Source: CAD feature listing. Evaluate the final solid. Frame: model axes, mm. A direction names the side the tool comes from. Coordinates: 2 decimals unless noted, no trailing zeros. Write each loop counter-clockwise with the first axis right and the second up, starting at its lowest first coordinate (ties: lowest second). Pieces come first, ordered by that corner, then holes. Notation, with made-up numbers: (-13.5, 45) -> (23.5, 45) arc R26 ccw to (23.5, 60) -> close; hole circle Ø2 at (17.5, 11.25). An arc over 180 degrees is marked (long way). One line per item, written item: value. Start each with the question number.
1. First-contact query: P1, Ø3, axis at x = -13, y = -54.5, coming from the -Z side; P2, Ø8.5, axis at y = -38, z = -12.5, coming from the +X side; P3, Ø6, axis at y = -34.5, z = -4, coming from the +X side. Flat tips, straight axial feed; report the tip coordinate or a pass-through.
2. Access query for faces 3 (the cylindrical face through (-32.22, -31.29, 0.51)), 4 (the flat face through (-29, -56.5, -8)). Directions: +Z, -Z, +X, -X, +Y, -Y. A direction counts if a zero-diameter tool reaches every point of the face in a straight line with its end or side. Return the directions, or none.
3. Mould query, pull axis X, two halves, no side actions, for faces 1 (the flat face through (-29, 1, -17)), 2 (the cylindrical face through (-0.86, -55.6, -8.62)). Classes: released by +X, released by -X, zero draft, split by the parting line, or undercut.
4. Line query: line 1 (Y direction, x = -28.25, z = 0.55); line 2 (Z direction, x = -35, y = -31); line 3 (X direction, y = -18, z = -9.25). Output: solid intervals per line, ascending.
5. Section query D-D, the plane x = -51.5. Output: boundary loops of the cut face in (y, z), and give its area (3 significant figures).
6. Section query C-C, the plane y = -55.5. Output: boundary loops of the cut face in (x, z), and give its area (3 significant figures).
7. Section query B-B, the plane z = -1. Output: boundary loops of the cut face in (x, y).
8. Section query A-A, the plane x = -28.25. Output: boundary loops of the cut face in (y, z).
from build123d import *

# Parameters (mm, degrees)
F0_W     = 60
F0_H     = 60
F0_W_2   = 56.5
F0_H_2   = 56.5
F1_DEPTH = 17
F2_DEPTH = 1
F3_DEPTH = 17
F4_R     = 5
F5_DEPTH = 25
F6_R     = 3


with BuildPart() as f1:
    # F0 (on Top) → F1 (new body)
    with BuildSketch(Plane.XY):
        with Locations((-28.25, -28.25)):
            Rectangle(F0_W, F0_H)
        with Locations((-28.25, -28.25)):
            Rectangle(F0_W_2, F0_H_2, mode=Mode.SUBTRACT)
    extrude(amount=-F1_DEPTH)

    # F0 (on Top) → F2 (join)
    with BuildSketch(Plane.XY):
        with Locations((-28.25, -28.25)):
            Rectangle(F0_W, F0_H)
        with Locations((-28.25, -28.25)):
            Rectangle(F0_W_2, F0_H_2, mode=Mode.SUBTRACT)
        with BuildLine():
            ThreePointArc((1.75, 1.75), (-28.25, 14.176407), (-58.25, 1.75))
            Line((-58.25, 1.75), (1.75, 1.75))
        make_face()
        with BuildLine():
            Line((1.75, 1.75), (1.75, -58.25))
            ThreePointArc((1.75, -58.25), (10.946889, -44.485883), (14.176407, -28.25))
            ThreePointArc((14.176407, -28.25), (10.946889, -12.014117), (1.75, 1.75))
        make_face()
        with BuildLine():
            Line((1.75, -58.25), (-58.25, -58.25))
            ThreePointArc((-58.25, -58.25), (-28.25, -70.676407), (1.75, -58.25))
        make_face()
        with BuildLine():
            ThreePointArc((-58.25, 1.75), (-70.676407, -28.25), (-58.25, -58.25))
            Line((-58.25, -58.25), (-58.25, 1.75))
        make_face()
        with Locations((-28.25, -28.25)):
            Rectangle(F0_W_2, F0_H_2)
    extrude(amount=F2_DEPTH)

    # F0 (on Top) → F3 (join)
    with BuildSketch(Plane.XY):
        with BuildLine():
            ThreePointArc((1.75, 1.75), (-28.25, 14.176407), (-58.25, 1.75))
            Line((-58.25, 1.75), (1.75, 1.75))
        make_face()
        with BuildLine():
            ThreePointArc((-58.25, 1.75), (-70.676407, -28.25), (-58.25, -58.25))
            Line((-58.25, -58.25), (-58.25, 1.75))
        make_face()
        with BuildLine():
            Line((1.75, 1.75), (1.75, -58.25))
            ThreePointArc((1.75, -58.25), (10.946889, -44.485883), (14.176407, -28.25))
            ThreePointArc((14.176407, -28.25), (10.946889, -12.014117), (1.75, 1.75))
        make_face()
        with BuildLine():
            Line((1.75, -58.25), (-58.25, -58.25))
            ThreePointArc((-58.25, -58.25), (-28.25, -70.676407), (1.75, -58.25))
        make_face()
    extrude(amount=-F3_DEPTH)

    # F4 (on face) → F5 (cut)
    with BuildSketch(Plane.XY.offset(1)):
        with Locations((-28.25, -28.25)):
            Circle(F4_R)
    extrude(amount=-F5_DEPTH, mode=Mode.SUBTRACT)

    # F6
    f6_edges = [f1.edges().sort_by_distance(p)[0] for p in [
        (0, 0, -8.5),
        (-56.5, 0, -8.5),
        (-56.5, -56.5, -8.5),
        (0, -56.5, -8.5),
    ]]
    fillet(f6_edges, radius=F6_R)


solid = f1.part
Computed values:
1. P1: stops at z = 0
1. P2: stops at x = 13.82
1. P3: stops at x = 14.05
2. face 3: +Z, -Z
2. face 4: -Z
3. face 1: zero draft
3. face 2: undercut
4. line 1: y = -70.68 to -33.25, -23.25 to 14.18
4. line 2: z = 0 to 1
4. line 3: x = -69.42 to -56.5, 0 to 12.92
5. outline: (-63.74, -17) -> (-56.5, -17) -> (-56.5, 0) -> (0, 0) -> (0, -17) -> (7.24, -17) -> (7.24, 1) -> (-63.74, 1) -> close
5. area: 317 mm²
6. outline: (-60.77, -17) -> (-55.74, -17) -> (-55.74, 0) -> (-0.76, 0) -> (-0.76, -17) -> (4.27, -17) -> (4.27, 1) -> (-60.77, 1) -> close
6. area: 236 mm²
7. outline: circle Ø84.85 at (-28.25, -28.25); hole (-56.5, -53.5) arc R3 ccw to (-53.5, -56.5) -> (-3, -56.5) arc R3 ccw to (0, -53.5) -> (0, -3) arc R3 ccw to (-3, 0) -> (-53.5, 0) arc R3 ccw to (-56.5, -3) -> close
8. outline: (-70.68, -17) -> (-56.5, -17) -> (-56.5, 0) -> (-33.25, 0) -> (-33.25, 1) -> (-70.68, 1) -> close; (-23.25, 0) -> (0, 0) -> (0, -17) -> (14.18, -17) -> (14.18, 1) -> (-23.25, 1) -> close
